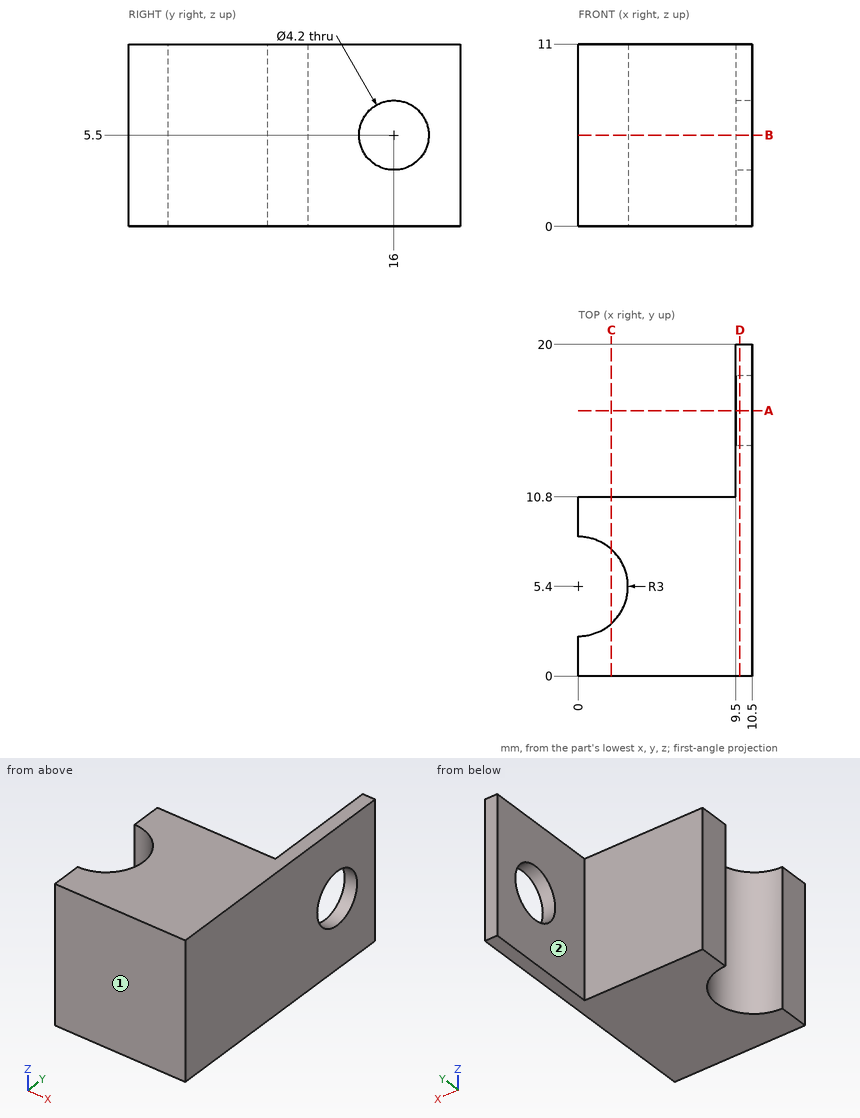
The figure shows three views and two pictorial views of one solid part (mm, origin at its lowest corner). Answer the questions. A direction names the side the tool comes from. Give positions to 0.01 mm unless a question says otherwise; leave off trailing zeros. Order: outer loops, then holes, each group sorted by start corner. A loop starts at its lowest first (then second) coordinate and runs counter-clockwise, first axis right, second up. Notation, with made-up numbers: (36, -8) -> (46, -8) arc R34 cw to (46, 27) -> close; hole circle Ø8 at (-20, 1.5). An arc over 180 degrees is marked (long way). Answer as CSV lines item,"result". Start each with the question number.
(1) Which of the six approach directions +Z, -Z, +X, -X, +Y, -Y give full straight-line access (tool end or side, diameter ignored) to the marked faces 1 and 2?
(2) Consider line 1 along Y through (x, z) = (9.8, 5.5); line 2 along X through (y, z) = (19, 1); line 3 along Y through (x, z) = (8.5, 3.5). Determine where each line is inside the solid, lowest interval first.
(3) Section A-A, the plane y = 16 is taken. Write down the section's boundary in (x, z).
(4) Section C-C, the plane x = 2 is taken. Write down the section's boundary in (y, z).
(5) This flat-tipped pin is pushed along its axis until it touches: pin 1 Ø5 at (x, z) = (9.5, 3.5) entering from -Y. Where does it stop, or does it pass through?
(6) Section D-D, the plane x = 9.75 is taken. Write down the section's boundary in (y, z).
(7) Section B-B, the plane z = 5.5 is taken. Write down the section's boundary in (x, y).
Entries:
1,face 1,"+Z, -Z, +X, -X, -Y"
1,face 2,"+Z, -Z, -X, +Y"
2,line 1,"0 to 13.9, 18.1 to 20"
2,line 2,"9.5 to 10.5"
2,line 3,"0 to 10.8"
3,outline,"(9.5, 0) -> (10.5, 0) -> (10.5, 3.4) -> (9.5, 3.4) -> close; (9.5, 7.6) -> (10.5, 7.6) -> (10.5, 11) -> (9.5, 11) -> close"
4,outline,"(0, 0) -> (3.16, 0) -> (3.16, 11) -> (0, 11) -> close; (7.64, 0) -> (10.8, 0) -> (10.8, 11) -> (7.64, 11) -> close"
5,pin 1,"y = 0"
6,outline,"(0, 0) -> (20, 0) -> (20, 11) -> (0, 11) -> close; hole circle Ø4.2 at (16, 5.5)"
7,outline,"(0, 0) -> (10.5, 0) -> (10.5, 13.9) -> (9.5, 13.9) -> (9.5, 10.8) -> (0, 10.8) -> (0, 8.4) arc R3 cw to (0, 2.4) -> close; (9.5, 18.1) -> (10.5, 18.1) -> (10.5, 20) -> (9.5, 20) -> close"
